from build123d import *

# Parameters (mm, degrees)
BOSS_EXTRUDE1_DEPTH      = 20.965
BOSS_EXTRUDE1_DEPTH_BACK = 20.965
F_4_CLEARANCE_HOLE1_D    = 3.2639
CUT_EXTRUDE1_DEPTH       = 2
SKETCH7_R                = 3.75
CUT_EXTRUDE2_DEPTH       = 2


with BuildPart() as part:
    # Sketch1 → Boss-Extrude1 (new, two sides: drawn at the far end of the back side and taken through both)
    with BuildSketch(Plane.XY.offset(-BOSS_EXTRUDE1_DEPTH_BACK)):
        Polygon((0, 50), (0, 0), (24.5, 0), (24.5, 2), (2, 2), (2, 50), align=None)
    extrude(amount=BOSS_EXTRUDE1_DEPTH + BOSS_EXTRUDE1_DEPTH_BACK)

    # #4 Clearance Hole1 (through all)
    with Locations(Plane(origin=(2, 0, 0), x_dir=(0, 0, -1), z_dir=(1, 0, 0))):
        with Locations((0, 44), (-14.722431864, 18.5), (14.722431864, 18.5)):
            Hole(F_4_CLEARANCE_HOLE1_D / 2)

    # Sketch6 → Cut-Extrude1 (cut)
    with BuildSketch(Plane(origin=(0, 2, 0), x_dir=(1, 0, 0), z_dir=(0, 1, 0))):
        with BuildLine():
            Line((11, -20.965), (11, -15.965))
            ThreePointArc((11, -15.965), (14.5, -12.465), (18, -15.965))
            Line((18, -15.965), (18, -20.965))
            ThreePointArc((18, -20.965), (14.5, -24.465), (11, -20.965))
        make_face()
    cut_extrude1 = extrude(amount=-CUT_EXTRUDE1_DEPTH, mode=Mode.SUBTRACT)

    # Mirror1: Cut-Extrude1 across plane
    add(cut_extrude1.mirror(Plane.XY), mode=Mode.SUBTRACT)

    # Sketch7 → Cut-Extrude2 (cut)
    with BuildSketch(Plane(origin=(2, 0, 0), x_dir=(0, 0, -1), z_dir=(1, 0, 0))):
        with Locations((0, 13)):
            Circle(SKETCH7_R)
    extrude(amount=-CUT_EXTRUDE2_DEPTH, mode=Mode.SUBTRACT)


solid = part.part
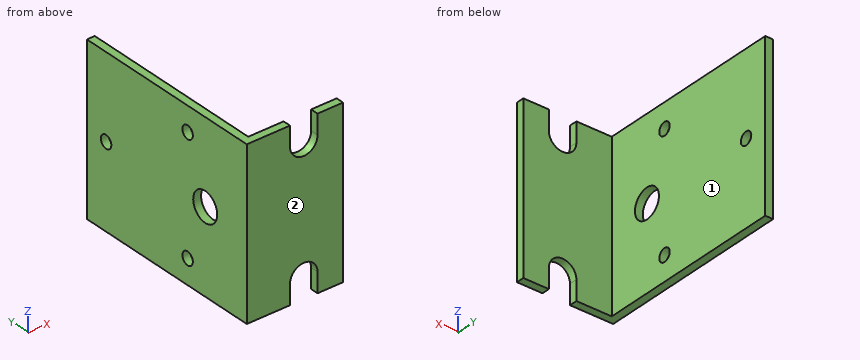
Source: CAD feature listing. Evaluate the final solid. Frame: model axes, mm. Face numbers are marked on the shaded views. A direction names the side the tool comes from. Give positions to 0.01 mm unless a question says otherwise; leave off trailing zeros. Write each loop counter-clockwise with the first axis right and the second up, starting at its lowest first coordinate (ties: lowest second). Pieces come first, ordered by that corner, then holes. Notation, with made-up numbers: (71.25, 80) -> (129.25, 80) arc R26 cw to (129.25, 107) -> close; hole circle Ø8 at (-17, -22.5). An arc over 180 degrees is marked (long way). Write item = value, one per line.
Q1. Cut plane C-C on y = 44. Return loops of the section in (x, z) (3 decimals), then the cut area to 3 significant figures.
Here are the results:
outline = (0, -20.965) -> (2, -20.965) -> (2, -1.632) -> (0, -1.632) -> close; (0, 1.632) -> (2, 1.632) -> (2, 20.965) -> (0, 20.965) -> close
area = 77.3 mm²
Q2. Line query: line 1 (Y direction, x = 1.25, z = 0); line 2 (X direction, y = 20.5, z = -13.5). Output: solid intervals per line, ascending. Write a range as from..to.
Here are the results:
line_1 = 0..9.25, 16.75..42.37, 45.63..50
line_2 = 0..2
Q3. Cut plane D-D on z = -9. Return loops of the section in (x, y).
Here are the results:
outline = (0, 0) -> (24.5, 0) -> (24.5, 2) -> (2, 2) -> (2, 50) -> (0, 50) -> close
Q4. Cut plane B-B on z = 0. Return loops of the section in (x, y), then the cut area to 3 significant figures.
Here are the results:
outline = (0, 0) -> (24.5, 0) -> (24.5, 2) -> (2, 2) -> (2, 9.25) -> (0, 9.25) -> close; (0, 16.75) -> (2, 16.75) -> (2, 42.37) -> (0, 42.37) -> close; (0, 45.63) -> (2, 45.63) -> (2, 50) -> (0, 50) -> close
area = 123 mm²
Q5. First-contact query: pin 1 (2.5 mm diameter, centred on y = 44, z = 0, fed in from -X); pin 2 (10 mm diameter, centred on x = 11.5, z = 15, fed in from +Y); pin 3 (12 mm diameter, centred on y = 17, z = 3.5, fed in from -X); pin 4 (4 mm diameter, centred on y = 19, z = 7, fed in from +X). Flat tips, straight axial feed; report the tip coordinate or a pass-through.
Here are the results:
pin_1 = through
pin_2 = 2
pin_3 = 0
pin_4 = 2
Q6. Cut plane A-A on y = 18.5. Return loops of the section in (x, z) (3 decimals), then the cut area to 3 significant figures.
Here are the results:
outline = (0, -20.965) -> (2, -20.965) -> (2, -16.354) -> (0, -16.354) -> close; (0, -13.09) -> (2, -13.09) -> (2, 13.09) -> (0, 13.09) -> close; (0, 16.354) -> (2, 16.354) -> (2, 20.965) -> (0, 20.965) -> close
area = 70.8 mm²
Q7. Reachability of the marked faces 1 and 2 from +Z, -Z, +X, -X, +Y, -Y: full face, straight path, thin tool, end or side. Return the list, or none.
Here are the results:
face_1 = +Z, -Z, +X, +Y
face_2 = +Z, -Z, +X, -X, -Y
